Could you check a few things on this model? Use its own coordinates, in mm. A direction names the side the tool comes from. Coordinates: 2 decimals unless noted, no trailing zeros. Loops run counter-clockwise (first coordinate to the right, second up) from the corner with the lowest first, then second, coordinate; pieces in that order, holes last.
1) Thinking about a two-plate mould opening in X: for faces 4 (the face through (-9, 0, 0)), 5 (the face through (9, 0, 0)), 6 (the face through (8.26, -4.444, 20.013)), 7 (the face through (0.105, -2.343, -17.847)), which applies, released by +X, released by -X, zero draft, split by the parting line, or undercut?
2) Imagine slicing it at D-D on z = -12. Please give me the cut outline in (x, y).
3) Imagine slicing it at B-B on y = 0. Please give me the cut outline in (x, z), plus the area to 3 significant figures.
4) Imagine slicing it at C-C on x = 5.75. Please give me the cut outline in (y, z).
5) Imagine slicing it at A-A on z = 0. Please give me the cut outline in (x, y).
6) For faces 1 (the face through (12, 13, 0)), 2 (the face through (-7.5, 1.4, 18.1)), 3 (the face through (10, 11, 0)), which set-ups out of +Z, -Z, +X, -X, +Y, -Y let a thin tool reach every point of the face, with its end or its side?
7) Will these pins go through, and if not, where does the flat tip stop? P1, Ø5, axis at x = -7, y = -4, coming from the +Z side; P2, Ø6, axis at x = -5, z = 12.5, coming from the -Y side; P3, Ø20.5, axis at y = -4, z = 9, coming from the +X side.
8) If I drill on line 1 along X through (y, z) = (9, -18); line 2 along X through (y, z) = (13.5, -6); line 3 along Y through (x, z) = (-7, 14), over which ranges is the centre line in solid material (lowest first)?
```python
from build123d import *

# Parameters (mm, degrees)
SKETCH2_R           = 2.5
BOSS_EXTRUDE1_DEPTH = 3


with BuildPart() as part:
    # Sketch1 → Revolve1 (revolve)
    with BuildSketch(Plane.XY):
        Polygon((9, 0), (-9, 0), (-9, 20.5), (-7.5, 20.5), (-7.5, 18), (7.5, 18), (7.5, 20.5), (9, 20.5), align=None)
    revolve(axis=Axis((9, 0, 0), (-1, 0, 0)))

    # Sketch2 → Boss-Extrude1 (add)
    with BuildSketch(Plane(origin=(9, 0, 0), x_dir=(0, 0, -1), z_dir=(1, 0, 0))):
        with Locations(Location((0, 13.5, 0), (0, 0, 90))):
            Circle(SKETCH2_R)
    extrude(amount=BOSS_EXTRUDE1_DEPTH)


solid = part.part
```
Filled in:
1. face 4: released by -X
1. face 5: released by +X
1. face 6: zero draft
1. face 7: undercut
2. outline: (-9, -16.62) - (-7.5, -16.62) - (-7.5, -13.42) - (7.5, -13.42) - (7.5, -16.62) - (9, -16.62) - (9, 16.62) - (7.5, 16.62) - (7.5, 13.42) - (-7.5, 13.42) - (-7.5, 16.62) - (-9, 16.62) - close
3. outline: (-9, -20.5) - (-7.5, -20.5) - (-7.5, -18) - (7.5, -18) - (7.5, -20.5) - (9, -20.5) - (9, 20.5) - (7.5, 20.5) - (7.5, 18) - (-7.5, 18) - (-7.5, 20.5) - (-9, 20.5) - close
3. area: 663 mm2
4. outline: circle Ø36 at (0, 0)
5. outline: (-9, -20.5) - (-7.5, -20.5) - (-7.5, -18) - (7.5, -18) - (7.5, -20.5) - (9, -20.5) - (9, 11) - (12, 11) - (12, 16) - (9, 16) - (9, 20.5) - (7.5, 20.5) - (7.5, 18) - (-7.5, 18) - (-7.5, 20.5) - (-9, 20.5) - close
6. face 1: +Z, -Z, +X, +Y, -Y
6. face 2: none
6. face 3: +X
7. P1: stops at z = 20.44
7. P2: stops at y = -17.4
7. P3: stops at x = 9
8. line 1: x = -9 to -7.5, 7.5 to 9
8. line 2: x = -9 to 9
8. line 3: y = -11.31 to 11.31
